Input: part model. Units: mm. Frame: model coordinates. A direction names the side the tool comes from. Round coordinates to 2 decimals unless told otherwise and drop trailing zeros. Loops run counter-clockwise (first coordinate to the right, second up) from the corner with the lowest first, then second, coordinate; pieces in that order, holes last. Notation, with made-up numbers: M 44.25,-26 L 88.25,-26 A3 ccw 88.25,-21 Z; hole C -17,0.25 d10. An arc over 180 degrees is marked long. Put each result on its own line as item: value. Start each with the question number.
1) Section B-B on z = 16. Output: boundary loops of the cut face in (x, y), plus the area to 3 significant figures.
2) Section A-A on y = 4.96. Output: boundary loops of the cut face in (x, z), plus the area to 3 significant figures.
3) Reachability of faces 4 (the face through (-1, 41, 3.208)), 5 (the face through (-1, -41, 23.148)), 6 (the face through (-1, 40, 24)), 7 (the face through (-1, -40, -2)) from +Z, -Z, +X, -X, +Y, -Y: full face, straight path, thin tool, end or side. Return the list, or none.
4) Section D-D on z = -1.5. Output: boundary loops of the cut face in (x, y).
5) Line query: probe 1 along Z at (x, y) = (-0.75, 4.96); probe 2 along Z at (x, y) = (-2.7, 0); probe 3 along Y at (x, z) = (-0.2, 6). Output: solid intervals per line, ascending.
6) Draft query along Z for faces 1 (the face through (-1, 1, 25.208)), 2 (the face through (-1.48, -6.03, 13.69)), 3 (the face through (-1, -42, 3.208)). Return one class per face: +Z half, -Z half, draft (parallel to the pull), parting line (faces both ways), or undercut.
7) Section C-C on x = -2.35. Output: boundary loops of the cut face in (y, z), plus the area to 3 significant figures.
8) Pin query (flat end, axial travel): pin 1 (1.6 mm diameter, centred on x = -2, z = 24, fed in from -Y); pin 2 (1.5 mm diameter, centred on x = -1, z = -3, fed in from +Y); pin 3 (0.9 mm diameter, centred on x = -1.5, y = 41.5, fed in from +Z). Return the tip coordinate at first contact, or that it passes through.
Solid Edge part; units mm, degrees
sketch "Sketch1" plane through (0, 0, 0) normal (1, 0, 0) x (0, 1, 0)
  circle A0 centre (4.96, 13.2085) radius 11
  line L0 (40, -6.7915) -> (40, 3.2085)
  line L1 (40, 3.2085) -> (43, 3.2085)
  line L2 (43, 3.2085) -> (43, 23.1485)
  line L3 (43, 23.1485) -> (40, 23.1485)
  line L4 (40, 23.1485) -> (40, 25.2085)
  line L5 (40, 25.2085) -> (-40, 25.2085)
  line L6 (-40, 25.2085) -> (-40, 23.1485)
  line L7 (-40, 23.1485) -> (-43, 23.1485)
  line L8 (-43, 23.1485) -> (-43, 3.2085)
  line L9 (-43, 3.2085) -> (-40, 3.2085)
  line L10 (-40, 3.2085) -> (-40, -6.7915)
  line L11 (-40, -6.7915) -> (40, -6.7915)
  dimension "D1" = 43
  dimension "D2" = 40
  dimension "D3" = 40
  dimension "D4" = 40
extrude "Protrusion1" add sketch "Sketch1" against normal blind 3
properties material "Acier"
Geometry results:
1. outline: M -3,-43 L 0,-43 L 0,-5.68 L -3,-5.68 Z; M -3,15.6 L 0,15.6 L 0,43 L -3,43 Z
1. area: 194 mm²
2. outline: M -3,-6.79 L 0,-6.79 L 0,2.21 L -3,2.21 Z; M -3,24.21 L 0,24.21 L 0,25.21 L -3,25.21 Z
2. area: 30.0 mm²
3. face 4: -Z, +X, -X, +Y
3. face 5: +Z, +X, -X, -Y
3. face 6: +Z, +X, -X, +Y
3. face 7: -Z, +X, -X, -Y
4. outline: M -3,-40 L 0,-40 L 0,40 L -3,40 Z
5. probe 1: z = -6.79 to 2.21, 24.21 to 25.21
5. probe 2: z = -6.79 to 3.39, 23.03 to 25.21
5. probe 3: y = -43 to -3.35, 13.27 to 43
6. face 1: +Z half
6. face 2: undercut
6. face 3: -Z half
7. outline: M -43,3.21 L -40,3.21 L -40,-6.79 L 40,-6.79 L 40,3.21 L 43,3.21 L 43,23.15 L 40,23.15 L 40,25.21 L -40,25.21 L -40,23.15 L -43,23.15 Z; hole C 4.96,13.21 d22
7. area: 2,300 mm²
8. pin 1: stops at y = -40
8. pin 2: stops at y = 40
8. pin 3: stops at z = 23.15
